```python
from build123d import *

# Parameters (mm, degrees)
F0_R     = 9.525
F1_DEPTH = 6.35
F2_DEPTH = 38.1


with BuildPart() as f1:
    # F0 (on Front) → F1 (new body)
    with BuildSketch(Plane.XZ):
        Polygon((-10.77674, 101.6), (-47.625, 101.6), (-84.47326, 101.6), (-109.903924, 13.530285), (-104.817793, -22.708416), (9.567793, -22.708416), (14.653924, 13.530285), align=None)
        with Locations((-95.25, 0)):
            Circle(F0_R, mode=Mode.SUBTRACT)
        Circle(F0_R, mode=Mode.SUBTRACT)
        with BuildLine():
            ThreePointArc((-34.925, 73.292352), (-38.644744, 64.312096), (-47.625, 60.592352))
            ThreePointArc((-47.625, 60.592352), (-60.325, 73.292352), (-47.625, 85.992352))
            ThreePointArc((-47.625, 85.992352), (-38.644744, 82.272608), (-34.925, 73.292352))
        make_face(mode=Mode.SUBTRACT)
    extrude(amount=F1_DEPTH)

    # F0 (on Front) → F2 (join)
    with BuildSketch(Plane.XZ):
        with Locations((-95.25, 0)):
            Circle(F0_R)
        Circle(F0_R)
    extrude(amount=F2_DEPTH)


solid = f1.part
```
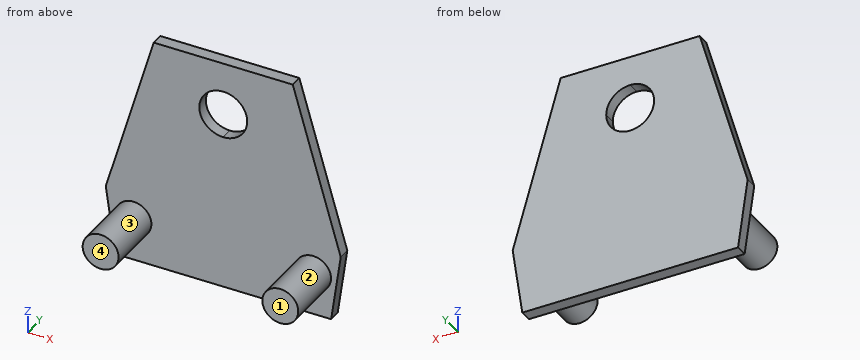
Part model, mm, in its own coordinate system. Face numbers are marked on the shaded views. A direction names the side the tool comes from. Round coordinates to 2 decimals unless told otherwise and drop trailing zeros. Loops run counter-clockwise (first coordinate to the right, second up) from the corner with the lowest first, then second, coordinate; pieces in that order, holes last. Notation, with made-up numbers: (30, 40) -> (63, 40) arc R31 ccw to (63, 70) -> close; hole circle Ø5 at (21.25, 69.25). An arc over 180 degrees is marked (long way). Use one line per item in the form item = value. Start each with the question number.
Item 1: Two-plate mould, pull along X, no slides. Class the marked faces 1 and 2: released by +X, released by -X, zero draft, split by the parting line, or undercut.
Item 2: Band-saw the part on D-D (x = -73). List the corners of the cut face in (y, z), plus the area to 3 significant figures.
Item 3: Drill centre lines: line 1 along X through (y, z) = (-24, 2); line 2 along X through (y, z) = (-35.5, -5); line 3 along Y through (x, z) = (-76, 13.5). Where is each one in solid material? Low to high.
Item 4: Tool access for the marked faces 3 and 4: list every direction of +Z, -Z, +X, -X, +Y, -Y with a clear straight run to the whole face (end or side of a thin tool).
Item 5: Band-saw the part on B-B (y = -17.5). List the corners of the cut face in (x, z) (3 decimals).
Item 6: Drop flat-ended pins along their axis: pin 1 Ø1.5 at (x, z) = (-91, 74) entering from -Y; pin 2 Ø12 at (x, y) = (-12.5, -12.5) entering from -Z. Give the stop position or say it passes through.
Item 7: Band-saw the part on A-A (x = -39.5). List the corners of the cut face in (y, z).
Item 8: Band-saw the part on C-C (z = 0). List the corners of the cut face in (x, y) (3 decimals), plus the area to 3 significant figures.
Data:
q1.face_1 = zero draft
q1.face_2 = undercut
q2.outline = (-6.35, -22.71) -> (0, -22.71) -> (0, 101.6) -> (-6.35, 101.6) -> close
q2.area = 789 mm^2
q3.line_1 = -104.56 to -85.94, -9.31 to 9.31
q3.line_2 = -103.36 to -87.14, -8.11 to 8.11
q3.line_3 = -6.35 to 0
q4.face_3 = -Y
q4.face_4 = +Z, -Z, +X, -X, -Y
q5.outline = circle Ø19.05 at (-95.25, 0); circle Ø19.05 at (0, 0)
q6.pin_1 = -6.35
q6.pin_2 = -6.96
q7.outline = (-6.35, -22.71) -> (0, -22.71) -> (0, 63.53) -> (-6.35, 63.53) -> close; (-6.35, 83.05) -> (0, 83.05) -> (0, 101.6) -> (-6.35, 101.6) -> close
q8.outline = (-108.005, -6.35) -> (-104.775, -6.35) -> (-104.775, -38.1) -> (-85.725, -38.1) -> (-85.725, -6.35) -> (-9.525, -6.35) -> (-9.525, -38.1) -> (9.525, -38.1) -> (9.525, -6.35) -> (12.755, -6.35) -> (12.755, 0) -> (-108.005, 0) -> close
q8.area = 1,980 mm^2
